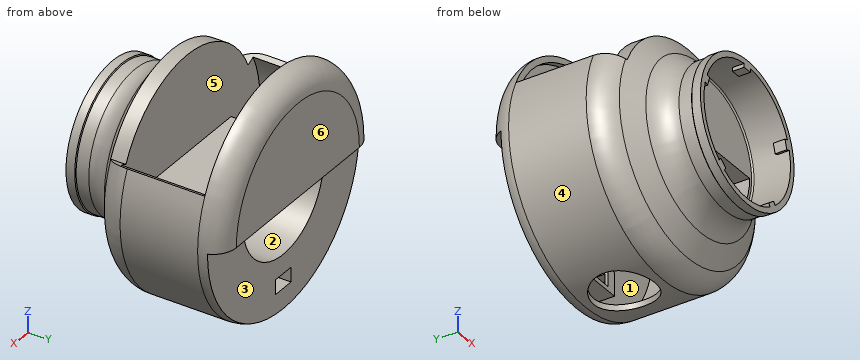
```python
from build123d import *

# Parameters (mm, degrees)
CUT_EXTRUDE3_DEPTH           = 60
CUT_EXTRUDE5_DEPTH           = 2
CUT_EXTRUDE5_DEPTH_BACK      = 30
SKETCH9_R                    = 38
SKETCH9_R_2                  = 23
SKETCH19_W                   = 12
SKETCH19_H                   = 36.5
CUT_REVOLVE2_ANGLE           = 65
CUT_REVOLVE2_OTHER_WAY_ANGLE = 65
SKETCH21_W                   = 3.25
SKETCH21_H                   = 4
BOSS_EXTRUDE3_DEPTH          = 1.35
CIRPATTERN1_COUNT            = 5
CUT_EXTRUDE9_START           = -5
CUT_EXTRUDE9_DEPTH           = 5
SKETCH23_R                   = 10.5
CUT_EXTRUDE10_DEPTH          = 10
SKETCH24_W                   = 15
SKETCH24_H                   = 8
BOSS_EXTRUDE4_DEPTH          = 8
SKETCH26_W                   = 8
SKETCH26_H                   = 5
CUT_EXTRUDE11_DEPTH          = 10
SKETCH27_W                   = 4
SKETCH27_H                   = 5
CUT_EXTRUDE12_DEPTH          = 5
CUT_EXTRUDE14_DEPTH          = 2
CUT_EXTRUDE14_DEPTH_BACK     = 30


# Read off the part's stored shape, not the designer's step: Cut-Extrude9
with BuildPart() as part:
    # Sketch1 → Revolve1 (revolve)
    with BuildSketch(Plane.XY, mode=Mode.PRIVATE) as revolve1_sk:
        with BuildLine():
            Line((0, 63.427876097), (32, 63.427876097))
            ThreePointArc((32, 63.427876097), (37.656854249, 61.084730346), (40, 55.427876097))
            Line((40, 55.427876097), (40, 28.846818009))
            ThreePointArc((40, 28.846818009), (38.792081772, 24.082439968), (35.460140376, 20.469057744))
            Line((35.460140376, 20.469057744), (28.539859624, 15.958818353))
            ThreePointArc((28.539859624, 15.958818353), (25.207918228, 12.345436129), (24, 7.581058088))
            Line((24, 7.581058088), (24, 3.25))
            Line((24, 3.25), (24.35, 3))
            Line((24.35, 3), (24.35, 0))
            Line((24.35, 0), (22.5, 0))
            Line((22.5, 0), (22.5, 12.5))
            ThreePointArc((22.5, 12.5), (22.353553391, 12.853553391), (22, 13))
            Line((22, 13), (0, 13))
            Line((0, 13), (0, 63.427876097))
        make_face()
    revolve(revolve1_sk.sketch.rotate(Axis((0, 0, 0), (0, 1, 0)), 90), axis=Axis((0, 0, 0), (0, 1, 0)))

    # Sketch11 → Cut-Extrude3 (cut)
    with BuildSketch(Plane(origin=(0, 13, 0), x_dir=(-1, 0, 0), z_dir=(0, -1, 0))):
        with BuildLine():
            Line((-21, 0), (21, 0))
            ThreePointArc((21, 0), (0, 21), (-21, 0))
        make_face()
    extrude(amount=-CUT_EXTRUDE3_DEPTH, mode=Mode.SUBTRACT)

    # Sketch9 → Cut-Extrude5 (cut, two sides: drawn at the far end of the back side and taken through both)
    with BuildSketch(Plane(origin=(0, 55.427876097, 0), x_dir=(1, 0, 0), z_dir=(0, 1, 0)).offset(-CUT_EXTRUDE5_DEPTH_BACK)):
        with Locations(Location((0, 0, 0), (0, 0, 270))):
            Circle(SKETCH9_R)
        with Locations(Location((0, 0, 0), (0, 0, 270))):
            Circle(SKETCH9_R_2, mode=Mode.SUBTRACT)
    extrude(amount=CUT_EXTRUDE5_DEPTH + CUT_EXTRUDE5_DEPTH_BACK, mode=Mode.SUBTRACT)

    # Sketch19 → Cut-Revolve2 (revolve, cut)
    with BuildSketch(Plane(origin=(0, 0, 0), x_dir=(0, 0, -1), z_dir=(1, 0, 0))):
        with Locations((-41.064715832, 37.177876097)):
            Rectangle(SKETCH19_W, SKETCH19_H)
    revolve(axis=Axis((0, 0, 0), (0, 1, 0)), revolution_arc=CUT_REVOLVE2_ANGLE, mode=Mode.SUBTRACT)

    # Sketch19 → Cut-Revolve2 other way (revolve, cut)
    with BuildSketch(Plane(origin=(0, 0, 0), x_dir=(0, 0, -1), z_dir=(1, 0, 0))):
        with Locations((-41.064715832, 37.177876097)):
            Rectangle(SKETCH19_W, SKETCH19_H)
    revolve(axis=Axis((0, 0, 0), (0, -1, 0)), revolution_arc=CUT_REVOLVE2_OTHER_WAY_ANGLE, mode=Mode.SUBTRACT)

    # Sketch21 → Boss-Extrude3 (add)
    with BuildSketch(Plane(origin=(0, 0, 22.5), x_dir=(-1, 0, 0), z_dir=(0, 0, -1))):
        with Locations((0, 2)):
            Rectangle(SKETCH21_W, SKETCH21_H)
    boss_extrude3 = extrude(amount=BOSS_EXTRUDE3_DEPTH)

    # CirPattern1: Boss-Extrude3 ×5 about axis
    cirpattern1_axis = Axis((0, 0, 0), (0, 1, 0))
    for i in range(1, CIRPATTERN1_COUNT):
        add(boss_extrude3.rotate(cirpattern1_axis, i * 360 / CIRPATTERN1_COUNT))

    # Cut-Extrude9 outline → Cut-Extrude9 (cut)
    with BuildSketch(Plane(origin=(0, 63.427876097, 0), x_dir=(1, 0, 0), z_dir=(0, 1, 0)).offset(CUT_EXTRUDE9_START)):
        with BuildLine():
            ThreePointArc((40, 0), (0, 40), (-40, 0))
            Line((-40, 0), (-21, 0))
            ThreePointArc((-21, 0), (0, 21), (21, 0))
            Line((21, 0), (40, 0))
        make_face()
    extrude(amount=CUT_EXTRUDE9_DEPTH, mode=Mode.SUBTRACT)

    # Sketch23 → Cut-Extrude10 (cut)
    with BuildSketch(Plane(origin=(0, 0, -40), x_dir=(-1, 0, 0), z_dir=(0, 0, -1))):
        with Locations((0, 42.137876097)):
            Circle(SKETCH23_R)
    extrude(amount=-CUT_EXTRUDE10_DEPTH, mode=Mode.SUBTRACT)

    # Sketch24 → Boss-Extrude4 (add)
    with BuildSketch(Plane(origin=(0, 58.427876097, 0), x_dir=(1, 0, 0), z_dir=(0, 1, 0))):
        with Locations((0, 30)):
            Rectangle(SKETCH24_W, SKETCH24_H)
    extrude(amount=-BOSS_EXTRUDE4_DEPTH)

    # Sketch26 → Cut-Extrude11 (cut)
    with BuildSketch(Plane(origin=(0, 58.427876097, 0), x_dir=(1, 0, 0), z_dir=(0, 1, 0))):
        with Locations((0, 30)):
            Rectangle(SKETCH26_W, SKETCH26_H)
    extrude(amount=-CUT_EXTRUDE11_DEPTH, mode=Mode.SUBTRACT)

    # Sketch27 → Cut-Extrude12 (cut)
    with BuildSketch(Plane(origin=(7.5, 0, 0), x_dir=(0, 0, -1), z_dir=(1, 0, 0))):
        with Locations((30, 53.927876097)):
            Rectangle(SKETCH27_W, SKETCH27_H)
    extrude(amount=-CUT_EXTRUDE12_DEPTH, mode=Mode.SUBTRACT)

    # Sketch28 → Cut-Extrude14 (cut, two sides: drawn at the far end of the back side and taken through both)
    with BuildSketch(Plane(origin=(0, 55.427876097, 0), x_dir=(1, 0, 0), z_dir=(0, 1, 0)).offset(-CUT_EXTRUDE14_DEPTH_BACK)):
        with BuildLine():
            Line((-22.912878475, -2), (22.912878475, -2))
            ThreePointArc((22.912878475, -2), (0, -23), (-22.912878475, -2))
        make_face()
    extrude(amount=CUT_EXTRUDE14_DEPTH + CUT_EXTRUDE14_DEPTH_BACK, mode=Mode.SUBTRACT)


solid = part.part
```
Geometry check sheet. Reference: the model listing, model coordinates, mm. Face numbers are marked on the shaded views. A direction names the side the tool comes from. Coordinates: 2 decimals unless noted, no trailing zeros. Loops run counter-clockwise (first coordinate to the right, second up) from the corner with the lowest first, then second, coordinate; pieces in that order, holes last. Notation, with made-up numbers: (29, -39.75) - (33, -39.75) arc R24 cw to (33, -3.75) - close; hole circle Ø6 at (-5, 0.5). An arc over 180 degrees is marked (long way). One line per item, written item: value. Start each with the question number.
(1) Tool access check on the marked faces 1, 2 and 3. Record the directions out of +Z, -Z, +X, -X, +Y, -Y that give a thin tool (end or side, any length) a straight path to the whole face; none if there is none.
(2) Mould release check, pull along Z, two halves, no side actions. Record for the marked faces 4, 5 and 6: released by +Z, released by -Z, zero draft, split by the parting line, or undercut.
(3) Cross-section at B-B on x = 0. Count the separate pieces of the cut face and the enclosed holes in it, plus the area to 3 significant figures.
(4) Material ranges on line 1 (Z direction, x = 2.5, y = 54); line 2 (X direction, y = 34.5, z = -10.5); line 3 (Y direction, x = 9, z = 22), recorded low to high. Write a range as [from, to].
(5) Depth check by flat-ended pin: P1, Ø5, axis at y = 32.5, z = -11.5, coming from the +X side; P2, Ø5, axis at y = 40.5, z = 17, coming from the +X side; P3, Ø22, axis at x = -4, z = 8.5, coming from the -Y side. Enter the tip coordinate at first touch or a pass-through.
(6) Cross-section at A-A on y = 48.5. Enter the section's corners in (x, z), plus the area to 3 significant figures.
Results below:
1. face 1: none
1. face 2: +Y, -Y
1. face 3: -Z, +X, -X, +Y
2. face 4: split by the parting line
2. face 5: undercut
2. face 6: zero draft
3. separate pieces: 3
3. enclosed holes: 0
3. area: 1,010 mm2
4. line 1: z = [-39.92, -37.92], [-34, -32.5], [-27.5, -26], [-22.86, -20.85], [0, 2]
4. line 2: x = [-38.6, -36.52], [-20.46, -18.19], [18.19, 20.46], [36.52, 38.6]
4. line 3: y = [0, 25.43], [57.43, 63.43]
5. P1: stops at x = 38.97
5. P2: stops at x = 37.28
5. P3: stops at y = 13
6. outline: (-36.25, 16.9) arc R40 ccw to (-8.35, -39.12) - (-8.35, -37.07) arc R38 cw to (-34.44, 16.06) - close; (-22.91, 2) arc R23 ccw (long way) to (22.91, 2) - close; (8.35, -39.12) arc R40 ccw to (36.25, 16.9) - (34.44, 16.06) arc R38 cw to (8.35, -37.07) - close; hole (-21, 0) arc R21 ccw to (21, 0) - close
6. area: 510 mm2
